Autodesk Inventor part; units mm, degrees
ref_plane "YZ Plane" through (0, 0, 0) normal (1, 0, 0) x (0, 1, 0)
ref_plane "XZ Plane" through (0, 0, 0) normal (0, 1, 0) x (-1, 0, 0)
ref_plane "XY Plane" through (0, 0, 0) normal (0, 0, 1) x (1, 0, 0)
sketch "Sketch1" plane through (0, 0, 0) normal (0, 0, 1) x (1, 0, 0)
  line L0 (0, 0) -> (8, 0)
  line L1 (8, 0) -> (8, 10)
  line L2 (8, 10) -> (0, 10)
  line L3 (0, 10) -> (0, 0)
  dimension "d0" = 8
  dimension "d1" = 10
extrude "Extrusion1" add sketch "Sketch1" along normal blind 15
sketch "Sketch2" plane through (0, 0, 15) normal (0, 0, 1) x (1, 0, 0)
  line L0 (8, 10) -> (0, 10)
  line L1 (2.5, 10) -> (5.5, 10)
  line L2 (5.5, 10) -> (5.5, 3.5)
  line L3 (5.5, 3.5) -> (2.5, 3.5)
  line L4 (2.5, 3.5) -> (2.5, 10)
  line L5 (0, 10) -> (0, 0)
  line L6 (8, 0) -> (8, 10)
  line L7 (0, 0) -> (8, 0)
  dimension "d4" = 2.5
  dimension "d5" = 2.5
  dimension "d6" = 3.5
extrude "Extrusion2" cut sketch "Sketch2" against normal blind 15 contours L2 L3 L4 L0
fillet "Fillet2" radius 1 4 edges at (2.5, 10, 7.5) (5.5, 10, 7.5) (2.5, 3.5, 7.5) (5.5, 3.5, 7.5)
properties part number "koppelstuk"
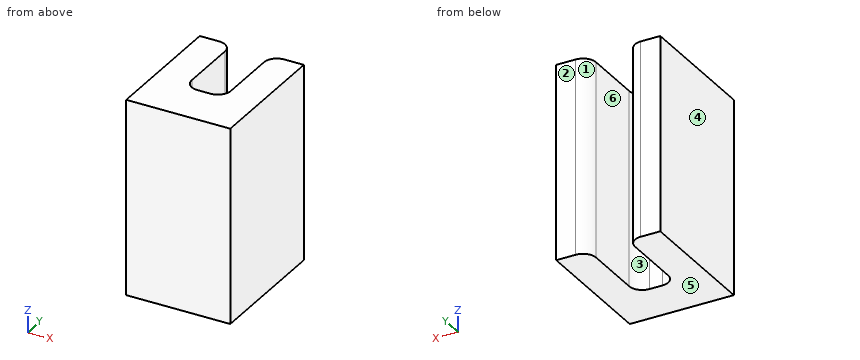
Design review of the part built by this model. Coordinates are the model's own, in mm. Face numbers are marked on the shaded views. A direction names the side the tool comes from. Coordinates: 2 decimals unless noted, no trailing zeros. Order: outer loops, then holes, each group sorted by start corner. A loop starts at its lowest first (then second) coordinate and runs counter-clockwise, first axis right, second up.
1) For the marked faces 1 and 2, list the 3-axis set-ups (+Z, -Z, +X, -X, +Y, -Y) from which the entire face can be reached by the end or side of a thin tool; tool diameter is ignored.
2) Take a section at B-B, the plane z = 12. Give the boundary of the cut face in (x, y).
3) Take a section at A-A, the plane y = 7. Give the boundary of the cut face in (x, z).
4) Take a section at C-C, the plane x = 4. Give the boundary of the cut face in (y, z).
5) Take a section at D-D, the plane y = 9.25. Give the boundary of the cut face in (x, z), and give its area (3 significant figures).
6) Clearance check with flat-ended pins moving along their axes: pin 1 (1.1 mm diameter, centred on x = 4, z = 11, fed in from +Y); pin 2 (3.5 mm diameter, centred on y = 7.5, z = 8.5, fed in from -X); pin 3 (1.5 mm diameter, centred on x = 2.5, z = 5.5, fed in from +Y). State where each tip first meets the part, or that it passes through.
7) Mouldability with a two-part tool opening along X and no side actions: class the marked faces 3, 4, 5 and 6 as +X half, -X half, draft (parallel to the pull), parting line (faces both ways), or undercut.
8) Wall thickness on line 1 along X through (y, z) = (7.5, 11); line 2 along X through (y, z) = (3.75, 1.5); line 3 along Y through (x, z) = (3.5, 7): over which ranges is each line inside the solid? List them lowest first.
Returned:
1. face 1: +Z, -Z, +Y
1. face 2: +Z, -Z, +X, -X, +Y
2. outline: (0, 0) - (8, 0) - (8, 10) - (6.5, 10) arc R1 ccw to (5.5, 9) - (5.5, 4.5) arc R1 cw to (4.5, 3.5) - (3.5, 3.5) arc R1 cw to (2.5, 4.5) - (2.5, 9) arc R1 ccw to (1.5, 10) - (0, 10) - close
3. outline: (0, 0) - (2.5, 0) - (2.5, 15) - (0, 15) - close; (5.5, 0) - (8, 0) - (8, 15) - (5.5, 15) - close
4. outline: (0, 0) - (3.5, 0) - (3.5, 15) - (0, 15) - close
5. outline: (0, 0) - (2.47, 0) - (2.47, 15) - (0, 15) - close; (5.53, 0) - (8, 0) - (8, 15) - (5.53, 15) - close
5. area: 74.0 mm2
6. pin 1: stops at y = 3.5
6. pin 2: stops at x = 0
6. pin 3: stops at y = 9.97
7. face 3: undercut
7. face 4: -X half
7. face 5: draft
7. face 6: undercut
8. line 1: x = 0 to 2.5, 5.5 to 8
8. line 2: x = 0 to 2.84, 5.16 to 8
8. line 3: y = 0 to 3.5
